```python
from build123d import *

# Parameters (mm, degrees)
F1_DEPTH  = 25.4
F2_T      = -2.54
F3_R      = 7.158021
F4_DEPTH  = 48.006
F5_R      = 5.120682
F11_DEPTH = 38.1
F10_R     = 5.120996
F12_DEPTH = 38.1
F9_R      = 5.158628
F13_DEPTH = 38.1
F7_R      = 5.120684
F14_DEPTH = 38.1
F6_R      = 5.005345
F15_DEPTH = 38.1
F8_R      = 4.585724
F16_DEPTH = 38.1


with BuildPart() as f1:
    # F0 (on Top) → F1 (new body)
    with BuildSketch(Plane.XY):
        Polygon((4.030147, -37.202981), (34.2338, -15.111281), (30.203654, 22.0917), (-4.030147, 37.202981), (-34.2338, 15.111281), (-30.203654, -22.0917), align=None)
    extrude(amount=F1_DEPTH)

    # F2
    f2_openings = [f1.faces().sort_by_distance(p)[0] for p in [
        (0, 0, 25.4),
    ]]
    offset(amount=F2_T, openings=f2_openings)

    # F3 (on Top) → F4 (join)
    with BuildSketch(Plane.XY):
        Circle(F3_R)
    extrude(amount=F4_DEPTH)

    # F5 (on Top) → F11 (join)
    with BuildSketch(Plane.XY):
        with Locations((28.946722, 20.595593)):
            Circle(F5_R)
    extrude(amount=F11_DEPTH)

    # F10 (on Top) → F12 (join)
    with BuildSketch(Plane.XY):
        with Locations((3.907301, -36.333404)):
            Circle(F10_R)
    extrude(amount=F12_DEPTH)

    # F9 (on Top) → F13 (join)
    with BuildSketch(Plane.XY):
        with Locations((32.073971, -14.988269)):
            Circle(F9_R)
    extrude(amount=F13_DEPTH)

    # F7 (on Top) → F14 (join)
    with BuildSketch(Plane.XY):
        with Locations((-32.698333, 13.326479)):
            Circle(F7_R)
    extrude(amount=F14_DEPTH)

    # F6 (on Top) → F15 (join)
    with BuildSketch(Plane.XY):
        with Locations((-29.656565, -21.907367)):
            Circle(F6_R)
    extrude(amount=F15_DEPTH)

    # F8 (on Top) → F16 (join)
    with BuildSketch(Plane.XY):
        with Locations((-4.096689, 34.406971)):
            Circle(F8_R)
    extrude(amount=F16_DEPTH)


solid = f1.part
```
Input: part model. Units: mm. Frame: model coordinates. A direction names the side the tool comes from. Round coordinates to 2 decimals unless told otherwise and drop trailing zeros. Write each loop counter-clockwise with the first axis right and the second up, starting at its lowest first coordinate (ties: lowest second). Pieces come first, ordered by that corner, then holes. Notation, with made-up numbers: (51.5, 67) -> (73.5, 67) arc R21 ccw to (73.5, 98) -> close; hole circle Ø2 at (64, 52.5). An arc over 180 degrees is marked (long way). Answer as CSV lines item,"result".
1. Ray query, L1, parallel to X at y = -5.5, z = 24; L2, parallel to X at y = -3.5, z = 11.5; L3, parallel to Z at x = -27.5, y = -8. Return the intervals inside material, ascending. Write a range as [from, to].
Geometry says:
L1,"x = [-32, -29.45], [-4.58, 4.58], [30.64, 33.19]"
L2,"x = [-32.22, -29.66], [-6.24, 6.24], [30.42, 32.98]"
L3,"z = [0, 2.54]"
2. Contact query for flat-ended pins moving along their axis: P1, Ø1.5, axis at y = -12.5, z = 36, coming from the +X side; P2, Ø11.5, axis at x = -30.5, y = 13.5, coming from the +Z side; P3, Ø2, axis at x = -21, y = -7.5, coming from the -Z side; P4, Ø9, axis at x = -15.5, y = 24, coming from the +Z side. Output: stop coordinate, or through.
Geometry says:
P1,"stops at x = 36.93"
P2,"stops at z = 38.1"
P3,"stops at z = 0"
P4,"stops at z = 25.4"
3. Section A-A (z = 22). Return the cut outline in (x, y).
Geometry says:
outline,"(-33.49, 8.27) -> (-30.75, -17.02) arc R5.01 ccw (long way) to (-25.25, -24.28) -> (-1.03, -34.97) arc R5.12 ccw (long way) to (8.45, -33.97) -> (28.87, -19.03) arc R5.16 ccw (long way) to (33.69, -10.09) -> (30.88, 15.85) arc R5.12 ccw (long way) to (25.35, 24.24) -> (0.41, 35.24) arc R4.59 ccw to (-8.65, 33.83) -> (-30.41, 17.91) arc R5.12 ccw (long way) to start; circle Ø14.32 at (0, 0); hole (-30.96, 8.51) -> (-28.19, -17.12) arc R5.01 cw to (-24.65, -21.77) -> (0.24, -32.76) arc R5.12 cw to (6.74, -32.07) -> (27.33, -17.01) arc R5.16 cw to (31.12, -9.92) -> (28.36, 15.51) arc R5.12 cw to (24.03, 22.04) -> (0.12, 32.6) arc R4.59 cw to (-7.6, 31.45) -> (-28.45, 16.19) arc R5.12 cw to start"
4. Section B-B (x = 20). Return the cut outline in (y, z).
Geometry says:
outline,"(-25.52, 0) -> (26.6, 0) -> (26.6, 25.4) -> (23.82, 25.4) -> (23.82, 2.54) -> (-22.38, 2.54) -> (-22.38, 25.4) -> (-25.52, 25.4) -> close"
5. Mould query, pull axis Y, two halves, no side actions, for faces 1 (the flat face through (0, 0, 48.006)), 2 (the cylindrical face through (33.677, 18.634, 18.783)). Classes: +Y half, -Y half, draft (parallel to the pull), parting line (faces both ways), or undercut.
Geometry says:
face 1,"draft"
face 2,"undercut"
6. Reachability of faces 3 (the flat face through (31, 3, 25.4)), 4 (the flat face through (-31, -4, 25.4)), 5 (the cylindrical face through (6.27, -40.877, 18.783)), 6 (the flat face through (29, 21, 38.1)), 7 (the flat face through (-4, 34, 38.1)) from +Z, -Z, +X, -X, +Y, -Y: full face, straight path, thin tool, end or side. Return the list, or none.
Geometry says:
face 3,"+Z, +X"
face 4,"+Z, -X"
face 5,"+Z"
face 6,"+Z, +X, -X, +Y, -Y"
face 7,"+Z, +X, -X, +Y"
7. Section D-D (y = 2.5). Return the cut outline in (x, z), plus the area to 3 significant figures.
Geometry says:
outline,"(-32.87, 0) -> (32.33, 0) -> (32.33, 25.4) -> (29.77, 25.4) -> (29.77, 2.54) -> (6.71, 2.54) -> (6.71, 48.01) -> (-6.71, 48.01) -> (-6.71, 2.54) -> (-30.31, 2.54) -> (-30.31, 25.4) -> (-32.87, 25.4) -> close"
area,"892 mm^2"
8. Section C-C (z = 36). Return the cut outline in (x, y), plus the area to 3 significant figures.
Geometry says:
outline,"circle Ø10.24 at (-32.7, 13.33); circle Ø10.01 at (-29.66, -21.91); circle Ø9.17 at (-4.1, 34.41); circle Ø14.32 at (0, 0); circle Ø10.24 at (3.91, -36.33); circle Ø10.24 at (28.95, 20.6); circle Ø10.32 at (32.07, -14.99)"
area,"636 mm^2"
